```python
from build123d import *

# Parameters (mm, degrees)
SKETCH_1_W                   = 26
SKETCH_1_H                   = 16
EXTRUDE_1_DEPTH              = 2
EXTRUDE_3_DEPTH              = 6
CUT_EXTRUDE_1_REACH          = 18.225
SKETCH_5_R                   = 1.4
EXTRUDE_4_REACH              = 29.427
SKETCH_6_W                   = 10
SKETCH_6_H                   = 0.5
CUT_EXTRUDE_2_REACH          = 29.427
SKETCH_7_W                   = 8
SKETCH_7_H                   = 0.5
HOLE_WIZARD_M2_1_D           = 2.1
HOLE_WIZARD_M2_1_CBORE_D     = 3.8
HOLE_WIZARD_M2_1_CBORE_DEPTH = 1
SKETCH_10_W                  = 1
SKETCH_10_H                  = 3.5
EXTRUDE_5_DEPTH              = 3.3
CHAMFER_1_SIZE               = 2
FILLET_2_R                   = 2
CUT_EXTRUDE_3_DEPTH          = 0.8


with BuildPart() as part:
    # ｽｹｯﾁ1 → ﾎﾞｽ - 押し出し1 (new body)
    with BuildSketch(Plane(origin=(0, 0, 0), x_dir=(1, 0, 0), z_dir=(0, 1, 0))):
        Rectangle(SKETCH_1_W, SKETCH_1_H)
    extrude(amount=EXTRUDE_1_DEPTH)

    # ｽｹｯﾁ4 → ﾎﾞｽ - 押し出し3 (add)
    with BuildSketch(Plane.XY.offset(8)):
        Polygon((-7, -3.5), (-4.5, -3.5), (-3, 0), (-7.9, 0), align=None)
        Polygon((3, 0), (4.5, -3.5), (7, -3.5), (7.9, 0), align=None)
    extrude(amount=-EXTRUDE_3_DEPTH)

    # ｽｹｯﾁ5 → ｶｯﾄ - 押し出し1 (cut, up to next)
    with BuildSketch(Plane(origin=(0, 2, 0), x_dir=(1, 0, 0), z_dir=(0, 1, 0)), mode=Mode.PRIVATE) as cut_extrude_1_sk1:
        with Locations(Location((0, -5, 0), (0, 0, 270))):
            Circle(SKETCH_5_R)
    cut_extrude_1_tool1 = extrude(cut_extrude_1_sk1.sketch, amount=-CUT_EXTRUDE_1_REACH, mode=Mode.PRIVATE) & part.part
    add(cut_extrude_1_tool1.solids().sort_by_distance((0, 2, 5))[0], mode=Mode.SUBTRACT)

    # ﾎﾞｽ - 押し出し4: up to this face of the body (flat: up to its plane)
    extrude_4_end = Plane(part.part.faces().sort_by_distance((-13, 1, 0))[0])
    # ｽｹｯﾁ6 → ﾎﾞｽ - 押し出し4 (add, up to the picked face)
    with BuildSketch(Plane(origin=(13, 0, 0), x_dir=(0, 0, -1), z_dir=(1, 0, 0)), mode=Mode.PRIVATE) as extrude_4_sk1:
        with Locations((3, -0.25)):
            Rectangle(SKETCH_6_W, SKETCH_6_H)
    extrude_4_tool1 = split(extrude(extrude_4_sk1.sketch, amount=-EXTRUDE_4_REACH, mode=Mode.PRIVATE), bisect_by=extrude_4_end, keep=Keep.BOTH, mode=Mode.PRIVATE)
    add(extrude_4_tool1.solids().sort_by(Axis((13, -0.25, -3), (-1, 0, 0)))[0])

    # ｽｹｯﾁ7 → ｶｯﾄ - 押し出し2 (cut, up to next)
    with BuildSketch(Plane(origin=(13, 0, 0), x_dir=(0, 0, -1), z_dir=(1, 0, 0)), mode=Mode.PRIVATE) as cut_extrude_2_sk1:
        with Locations((4, 1.75)):
            Rectangle(SKETCH_7_W, SKETCH_7_H)
    cut_extrude_2_tool1 = extrude(cut_extrude_2_sk1.sketch, amount=-CUT_EXTRUDE_2_REACH, mode=Mode.PRIVATE) & part.part
    add(cut_extrude_2_tool1.solids().sort_by_distance((13, 1.75, -4))[0], mode=Mode.SUBTRACT)

    # M2 丸平ねじ用座ぐり穴1 (through all)
    with Locations(Plane(origin=(0, 1.5, 0), x_dir=(1, 0, 0), z_dir=(0, 1, 0))):
        with Locations((10.5, 4)):
            hole_wizard_m2_1 = CounterBoreHole(HOLE_WIZARD_M2_1_D / 2, HOLE_WIZARD_M2_1_CBORE_D / 2, HOLE_WIZARD_M2_1_CBORE_DEPTH)

    # ｽｹｯﾁ10 → ﾎﾞｽ - 押し出し5 (add)
    with BuildSketch(Plane.XZ.offset(0.5)):
        with Locations((10.75, 0.25)):
            Rectangle(SKETCH_10_W, SKETCH_10_H)
    extrude_5 = extrude(amount=EXTRUDE_5_DEPTH)

    # ﾐﾗｰ1: M2 丸平ねじ用座ぐり穴1, ﾎﾞｽ - 押し出し5 across plane
    add(hole_wizard_m2_1.mirror(Plane(origin=(0, 0, 0), x_dir=(0, 0, 1), z_dir=(1, 0, 0))), mode=Mode.SUBTRACT)
    add(extrude_5.mirror(Plane(origin=(0, 0, 0), x_dir=(0, 0, 1), z_dir=(1, 0, 0))))

    # 面取り1
    # the kernel refuses this chamfer: 2 mm, written as the material it takes off along each edge
    with BuildSketch(Plane(origin=(18.143365976, 2, 8), x_dir=(0, 0.02749587661058627, -0.9996219169112968), z_dir=(-1, 0, 0))) as chamfer_1_piece_1:
        Polygon((CHAMFER_1_SIZE * 0.999621916911, CHAMFER_1_SIZE * 0.0274958766106), (-CHAMFER_1_SIZE * 0.0274958766106, CHAMFER_1_SIZE * 0.999621916911), (0, 0), align=None)
    extrude(amount=36.286731952, mode=Mode.SUBTRACT)

    # ﾌｨﾚｯﾄ2
    fillet_2_edges = [part.edges().sort_by_distance(p)[0] for p in [
        (13, 0.5, -8),
        (-13, 0.5, -8),
    ]]
    fillet(fillet_2_edges, radius=FILLET_2_R)

    # ｽｹｯﾁ12 → ｶｯﾄ - 押し出し3 (cut, symmetric)
    with BuildSketch(Plane.XY.offset(5)):
        Polygon((-7.9, 0), (-7, -3.5), (-6.4, -3.5), (-7.3, 0), align=None)
        Polygon((-3, 0), (-4.5, -3.5), (-5.1, -3.5), (-3.6, 0), align=None)
    cut_extrude_3 = extrude(amount=CUT_EXTRUDE_3_DEPTH, both=True, mode=Mode.SUBTRACT)

    # ﾐﾗｰ2: ｶｯﾄ - 押し出し3 across plane
    add(cut_extrude_3.mirror(Plane(origin=(0, 0, 0), x_dir=(0, 0, 1), z_dir=(1, 0, 0))), mode=Mode.SUBTRACT)


solid = part.part
```
Design review of the part built by this model. Coordinates are the model's own, in mm. A direction names the side the tool comes from. Give positions to 0.01 mm unless a question says otherwise; leave off trailing zeros. Order: outer loops, then holes, each group sorted by start corner. A loop starts at its lowest first (then second) coordinate and runs counter-clockwise, first axis right, second up. Notation, with made-up numbers: (15.5, -25.75) -> (49.5, -25.75) arc R24 ccw to (49.5, -1.75) -> close; hole circle Ø11 at (-10.75, -15). An arc over 180 degrees is marked (long way). Write item = value, one per line. Start each with the question number.
(1) Mouldability with a two-part tool opening along X and no side actions: class faces 4 (the face through (7, -2, 5.8)), 5 (the face through (11.521, 1.007, -5.602)), 6 (the face through (-7.456, -1.726, 3.115)) as +X half, -X half, draft (parallel to the pull), parting line (faces both ways), or undercut.
(2) For pin 1 (1.7 mm diameter, centred on x = 11.5, z = 4, fed in from -Y); pin 2 (1.2 mm diameter, centred on x = 5.5, z = 6.5, fed in from -Y); pin 3 (1.9 mm diameter, centred on x = -10.5, z = -3.5, fed in from +Y), all flat-tipped, find the tip position at first contact; note any pin that passes through.
(3) We need section A-A on z = -4. Write out the cut boundary in (x, y), plus the area to 3 significant figures.
(4) To check wall thickness, follow line 1 along Y through (x, z) = (-8, 1.75); line 2 along X through (y, z) = (1.25, 5); line 3 along Z through (x, y) = (-10.5, 1.3). State the ranges of each line that lie inside material, in increasing order.
(5) We need section B-B on x = -10.5. Write out the cut boundary in (y, z).
(6) For faces 1 (the face through (-11, -2, -1.5)), 2 (the face through (-4, -1.7, 5.8)), 3 (the face through (0, 1.5, -4)), list the 3-axis set-ups (+Z, -Z, +X, -X, +Y, -Y) from which the entire face can be reached by the end or side of a thin tool; tool diameter is ignored.
(7) We need section D-D on y = -3.25. State how many separate pieces and enclosed holes the cut face has, plus the area to 3 significant figures.
(8) We need section C-C on z = 5. Write out the cut boundary in (x, y).
Numbers:
q1.face_4 = draft
q1.face_5 = undercut
q1.face_6 = -X half
q2.pin_1 = 0
q2.pin_2 = -3.5
q2.pin_3 = 0.5
q3.outline = (-13, -0.5) -> (-11.55, -0.5) -> (-11.55, 0.5) -> (-12.4, 0.5) -> (-12.4, 1.5) -> (-13, 1.5) -> close; (-9.45, -0.5) -> (9.45, -0.5) -> (9.45, 0.5) -> (8.6, 0.5) -> (8.6, 1.5) -> (-8.6, 1.5) -> (-8.6, 0.5) -> (-9.45, 0.5) -> close; (11.55, -0.5) -> (13, -0.5) -> (13, 1.5) -> (12.4, 1.5) -> (12.4, 0.5) -> (11.55, 0.5) -> close
q3.area = 40.2 mm^2
q4.line_1 = -0.5 to 2
q4.line_2 = -13 to -1.4, 1.4 to 13
q4.line_3 = -8 to -5.9, -2.1 to 6.7
q5.outline = (-3.8, -1.5) -> (-0.5, -1.5) -> (-0.5, -2.95) -> (0.5, -2.95) -> (0.5, -2.1) -> (1.5, -2.1) -> (1.5, 0) -> (2, 0) -> (2, 6) -> (0, 8) -> (0, 2) -> (-3.8, 2) -> close; (-0.5, -8) -> (1.5, -8) -> (1.5, -5.9) -> (0.5, -5.9) -> (0.5, -5.05) -> (-0.5, -5.05) -> close
q6.face_1 = -Z, +X, -X, -Y
q6.face_2 = -Y
q6.face_3 = -Z, +X, -X, +Y
q7.separate_pieces = 4
q7.enclosed_holes = 0
q7.area = 35.2 mm^2
q8.outline = (-13, 0) -> (-7.3, 0) -> (-6.4, -3.5) -> (-5.1, -3.5) -> (-3.6, 0) -> (-1.4, 0) -> (-1.4, 2) -> (-13, 2) -> close; (1.4, 0) -> (3.6, 0) -> (5.1, -3.5) -> (6.4, -3.5) -> (7.3, 0) -> (13, 0) -> (13, 2) -> (1.4, 2) -> close
